CAD build for the part. Positions are in the model's coordinates, mm. A direction names the side the tool comes from. Round coordinates to 2 decimals unless told otherwise and drop trailing zeros. Loops run counter-clockwise (first coordinate to the right, second up) from the corner with the lowest first, then second, coordinate; pieces in that order, holes last. Notation, with made-up numbers: (-24.75, 86) -> (-0.75, 86) arc R29 ccw to (-0.75, 107) -> close; hole circle Ø4 at (24.5, 3). An arc over 180 degrees is marked (long way). Answer as CSV lines item,"result".
```python
from build123d import *

# Parameters (mm, degrees)
F0_W     = 7.62
F0_H     = 25.4
F1_DEPTH = 6.35
F3_DEPTH = 6.35
F4_R     = 2.286
F5_DEPTH = 7.62


with BuildPart() as f1:
    # F0 (on Top) → F1 (new body)
    with BuildSketch(Plane.XY):
        Rectangle(F0_W, F0_H)
    extrude(amount=F1_DEPTH)

    # F2 (on face) → F3 (cut, through all)
    with BuildSketch(Plane.XY.offset(6.35)):
        with BuildLine():
            ThreePointArc((-1.27, 6.604), (-0.195298, 0), (-1.27, -6.604))
            Line((-1.27, -6.604), (3.81, -6.604))
            Line((3.81, -6.604), (3.81, 6.604))
            Line((3.81, 6.604), (-1.27, 6.604))
        make_face()
    extrude(amount=-F3_DEPTH, mode=Mode.SUBTRACT)

    # F4 (on face) → F5 (cut, through all)
    with BuildSketch(Plane(origin=(-3.81, 0, 0), x_dir=(0, -1, 0), z_dir=(-1, 0, 0))):
        with Locations((-9.652, 3.175)):
            Circle(F4_R)
        with Locations((9.652, 3.175)):
            Circle(F4_R)
    extrude(amount=-F5_DEPTH, mode=Mode.SUBTRACT)


solid = f1.part
```
Q1. Slice it at A-A, the plane x = -0.75. Give the cut face in (y, z) (3 decimals).
Results:
outline,"(-12.7, 0) -> (-6.604, 0) -> (-6.604, 6.35) -> (-12.7, 6.35) -> close; (-4.775, 0) -> (4.775, 0) -> (4.775, 6.35) -> (-4.775, 6.35) -> close; (6.604, 0) -> (12.7, 0) -> (12.7, 6.35) -> (6.604, 6.35) -> close; hole circle Ø4.572 at (-9.652, 3.175); hole circle Ø4.572 at (9.652, 3.175)"
Q2. Slice it at D-D, the plane x = 3. Give the cut face in (y, z) (3 decimals).
Results:
outline,"(-12.7, 0) -> (-6.604, 0) -> (-6.604, 6.35) -> (-12.7, 6.35) -> close; (6.604, 0) -> (12.7, 0) -> (12.7, 6.35) -> (6.604, 6.35) -> close; hole circle Ø4.572 at (-9.652, 3.175); hole circle Ø4.572 at (9.652, 3.175)"
Q3. Two-plate mould, pull along Y, no slides. Class faces 3 (the flat face through (0, -12.7, 3)), 4 (the cylindrical face through (-0.196, 0.094, 3.219)), 5 (the flat face through (3.81, 12, 5)): pulls with the +Y half, pulls with the -Y half, needs draft (parallel to the pull), parting line crosses it, or undercut.
Results:
face 3,"pulls with the -Y half"
face 4,"undercut"
face 5,"needs draft"
Q4. Slice it at B-B, the plane y = 10.25. Give the cut face in (x, z), and give its area (3 significant figures).
Results:
outline,"(-3.81, 0) -> (3.81, 0) -> (3.81, 0.97) -> (-3.81, 0.97) -> close; (-3.81, 5.38) -> (3.81, 5.38) -> (3.81, 6.35) -> (-3.81, 6.35) -> close"
area,"14.8 mm2"
Q5. Tool access for faces 1 (the flat face through (1, -6.604, 3)), 2 (the cylindrical face through (-0.053, -11.832, 3.862)): list every direction of +Z, -Z, +X, -X, +Y, -Y with a clear straight run to the whole face (end or side of a thin tool).
Results:
face 1,"+Z, -Z, +X"
face 2,"+X, -X"
Q6. Slice it at C-C, the plane z = 4.5. Give the cut face in (x, y), and give its area (3 significant figures).
Results:
outline,"(-3.81, -12.7) -> (3.81, -12.7) -> (3.81, -11.51) -> (-3.81, -11.51) -> close; (-3.81, -7.79) -> (3.81, -7.79) -> (3.81, -6.6) -> (-1.27, -6.6) arc R20.83 ccw to (-1.27, 6.6) -> (3.81, 6.6) -> (3.81, 7.79) -> (-3.81, 7.79) -> close; (-3.81, 11.51) -> (3.81, 11.51) -> (3.81, 12.7) -> (-3.81, 12.7) -> close"
area,"79.2 mm2"
Q7. Drop a flat-ended pin along its axis: pin 1 Ø3 at (y, z) = (-9.5, 3.5) entering from +X. Give the stop position or say it passes through.
Results:
pin 1,"through"
Q8. Probe L1, parallel to Z at x = 3, y = 9.5; L2, parallel to Y at x = -1.75, z = 2; L3, parallel to Y at x = 0.75, z = 0.5. List the from-to ranges inside material, lowest first. Write a range as [from, to].
Results:
L1,"[0, 0.89], [5.46, 6.35]"
L2,"[-12.7, -11.61], [-7.69, 7.69], [11.61, 12.7]"
L3,"[-12.7, -6.6], [6.6, 12.7]"
